Verification items for the finished model (mm, model axes). A direction names the side the tool comes from. Round coordinates to 2 decimals unless told otherwise and drop trailing zeros. Write each loop counter-clockwise with the first axis right and the second up, starting at its lowest first coordinate (ties: lowest second). Pieces come first, ordered by that corner, then holes. Notation, with made-up numbers: (4, -35) - (45, -35) arc R19 ccw to (45, -20) - close; hole circle Ø2 at (-37.75, -3). An arc over 180 degrees is marked (long way). Answer as a JSON object with one key per item and string values.
Autodesk Inventor part; units mm, degrees
ref_plane "YZ Plane" through (0, 0, 0) normal (1, 0, 0) x (0, 1, 0)
ref_plane "XZ Plane" through (0, 0, 0) normal (0, 1, 0) x (-1, 0, 0)
ref_plane "XY Plane" through (0, 0, 0) normal (0, 0, 1) x (1, 0, 0)
sketch "Skizze1" plane through (0, 0, 0) normal (0, 0, 1) x (1, 0, 0)
  line L0 (-68.45, -44.2) -> (68.45, -44.2)
  line L1 (68.45, -44.2) -> (68.45, 44.2)
  line L2 (68.45, 44.2) -> (-68.45, 44.2)
  line L3 (-68.45, 44.2) -> (-68.45, -44.2)
  line L4 (-68.45, -44.2) -> (68.45, 44.2) construction
  line L5 (68.45, -44.2) -> (-68.45, 44.2) construction
  circle A0 centre (-63.75, -39) radius 1.375
  circle A1 centre (63.75, -39) radius 1.375
  circle A2 centre (63.75, 39) radius 1.375
  circle A3 centre (-63.75, 39) radius 1.375
  line L6 (0, 61.88) -> (0, -61.88)
  line L7 (-95.83, 0) -> (95.83, 0)
  circle A4 centre (-63.75, 31.5) radius 1.375
  circle A5 centre (-63.75, -31.5) radius 1.375
  line L8 (-63.75, 39) -> (-63.75, 31.5) construction
  circle A6 centre (-11.75, 0) radius 1.375
  point P0 (0, 0)
  dimension "d0" = 136.9
  dimension "d1" = 88.4
  dimension "d2" = 2.75
  dimension "d3" = 127.5
  dimension "d4" = 78
  dimension "d7" = 63
  dimension "d8" = 2.75
  dimension "d9" = 2.75
  dimension "d10" = 52
extrude "Extrusion1" add sketch "Skizze1" along normal blind 3.6 contours L3 L7 A6 L6 L0 | L6 L7 L1 L0 | L3 L2 L6 L7 A6 | L6 L2 L1 L7
sketch "Skizze2" plane through (0, 0, 0) normal (0, 0, -1) x (-1, 0, 0)
  circle A0 centre (63.75, -31.5) radius 1.375
  circle A1 centre (63.75, 31.5) radius 1.375
  circle A2 centre (11.75, 0) radius 1.375
  line L0 (67.05, -28.2) -> (60.45, -28.2)
  line L1 (60.45, -28.2) -> (60.45, -34.8)
  line L2 (60.45, -34.8) -> (67.05, -34.8)
  line L3 (67.05, -34.8) -> (67.05, -28.2)
  line L4 (67.05, -28.2) -> (60.45, -34.8) construction
  line L5 (60.45, -28.2) -> (67.05, -34.8) construction
  line L6 (67.05, 34.8) -> (60.45, 34.8)
  line L7 (60.45, 34.8) -> (60.45, 28.2)
  line L8 (60.45, 28.2) -> (67.05, 28.2)
  line L9 (67.05, 28.2) -> (67.05, 34.8)
  circle A3 centre (63.75, 31.5) radius 1.375
  line L10 (67.05, 34.8) -> (60.45, 28.2) construction
  line L11 (60.45, 34.8) -> (67.05, 28.2) construction
  line L12 (15.05, 3.3) -> (8.45, 3.3)
  line L13 (8.45, 3.3) -> (8.45, -3.3)
  line L14 (8.45, -3.3) -> (15.05, -3.3)
  line L15 (15.05, -3.3) -> (15.05, 3.3)
  line L16 (15.05, 3.3) -> (8.45, -3.3) construction
  line L17 (8.45, 3.3) -> (15.05, -3.3) construction
  point P0 (0, 0)
  dimension "d11" = 6.6
  dimension "d12" = 6.6
extrude "Extrusion2" [suppressed]
sketch "Skizze3" plane through (0, 0, 3.6) normal (0, 0, 1) x (1, 0, 0)
  circle A0 centre (-63.75, 31.5) radius 1.375
  circle A1 centre (-63.75, -31.5) radius 1.375
  circle A2 centre (-11.75, 0) radius 1.375
  line L0 (-63.75, 31.5) -> (-63.75, -31.5) construction
  line L1 (-95.83, 0) -> (95.83, 0)
  line L2 (-67.25, -27) -> (-60.25, -27)
  line L3 (-60.25, -27) -> (-60.25, 27)
  line L4 (-60.25, 27) -> (-67.25, 27)
  line L5 (-67.25, 27) -> (-67.25, -27)
  line L6 (-67.25, -27) -> (-60.25, 27) construction
  line L7 (-60.25, -27) -> (-67.25, 27) construction
  line L8 (-52.25, -34) -> (-43.25, -34)
  line L9 (-43.25, -34) -> (-43.25, -43)
  line L10 (-43.25, -43) -> (-52.25, -43)
  line L11 (-52.25, -43) -> (-52.25, -34)
  line L12 (-34.25, -34) -> (-25.25, -34)
  line L13 (-25.25, -34) -> (-25.25, -43)
  line L14 (-25.25, -43) -> (-34.25, -43)
  line L15 (-34.25, -43) -> (-34.25, -34)
  line L16 (-47.75, -34) -> (-47.75, -43) construction
  line L17 (-29.75, -34) -> (-29.75, -43) construction
  line L18 (-52.25, -38.5) -> (-43.25, -38.5) construction
  line L19 (-27.95, 22.5) -> (-7.95, 22.5)
  line L20 (-7.95, 22.5) -> (-7.95, 42.5)
  line L21 (-7.95, 42.5) -> (-27.95, 42.5)
  line L22 (-27.95, 42.5) -> (-27.95, 22.5)
  line L23 (-17.95, 42.5) -> (-17.95, 22.5) construction
  point P0 (0, 0)
  point P1 (-63.75, 0)
  dimension "d15" = 7
  dimension "d16" = 54
  dimension "d17" = 9
  dimension "d18" = 9
  dimension "d19" = 9
  dimension "d20" = 18
  dimension "d21" = 16
  dimension "d22" = 7
  dimension "d23" = 20
  dimension "d25" = 11
  dimension "d26" = 20
  dimension "d29" = 45.8
extrude "Extrusion3" cut sketch "Skizze3" against normal blind 3 contours L3 L2 L5 L1 | L1 L5 L4 L3 | L8 L9 L10 L11 | L12 L13 L14 L15 | L22 L21 L20 L19
sketch "Skizze4" plane through (0, 0, 3.6) normal (0, 0, 1) x (1, 0, 0)
  line L0 (-31.95, 18.5) -> (-17.75, 18.5)
  line L1 (-17.75, 18.5) -> (-17.75, -30)
  line L2 (-17.75, -30) -> (-56.25, -30)
  line L3 (-56.25, -30) -> (-56.25, 38.5)
  line L4 (-31.95, 18.5) -> (-31.95, 38.5)
  line L5 (-31.95, 38.5) -> (-56.25, 38.5)
  line L6 (-1.95, 35) -> (58.05, 35)
  line L7 (58.05, 35) -> (58.05, -35)
  line L8 (58.05, -35) -> (-1.95, -35)
  line L9 (-1.95, -35) -> (-1.95, 35)
  line L10 (-7.95, 22.5) -> (-27.95, 22.5)
  line L11 (-7.95, 42.5) -> (-7.95, 22.5)
  line L12 (-27.95, 42.5) -> (-7.95, 42.5)
  line L13 (-27.95, 22.5) -> (-27.95, 42.5)
  line L14 (-60.25, -27) -> (-67.25, -27)
  line L15 (-60.25, 27) -> (-60.25, -27)
  line L16 (-67.25, 27) -> (-60.25, 27)
  line L17 (-67.25, -27) -> (-67.25, 27)
  line L18 (-34.25, -34) -> (-25.25, -34)
  line L19 (-34.25, -43) -> (-34.25, -34)
  line L20 (-25.25, -43) -> (-34.25, -43)
  line L21 (-25.25, -34) -> (-25.25, -43)
  circle A0 centre (-11.75, 0) radius 1.375
  line L22 (-95.83, 0) -> (95.83, 0)
  line L23 (0, 61.88) -> (0, -61.88)
  point P0 (0, 0)
  dimension "d30" = 4
  dimension "d31" = 4
  dimension "d32" = 4
  dimension "d34" = 4
  dimension "d35" = 6
  dimension "d36" = 4
  dimension "d37" = 6
  dimension "d38" = 70
  dimension "d39" = 60
extrude "Extrusion4" cut sketch "Skizze4" against normal blind 2 contours L9 L6 L23 L22 | L22 L23 L8 L9 | L0 L1 L22 L3 L5 L4 | L1 L2 L3 L22 | L23 L6 L7 L22 | L22 L7 L8 L23
sketch "Skizze5" plane through (0, 0, 3.6) normal (0, 0, 1) x (1, 0, 0)
  circle A0 centre (-63.75, 39) radius 1.375
  circle A1 centre (-63.75, -39) radius 1.375
  circle A2 centre (63.75, -39) radius 1.375
  circle A3 centre (63.75, 39) radius 1.375
  line L0 (-67.25, 43) -> (-60.25, 43)
  line L1 (-60.25, 43) -> (-60.25, 36)
  line L2 (-60.25, 36) -> (-67.25, 36)
  line L3 (-67.25, 36) -> (-67.25, 43)
  line L4 (-67.25, -43) -> (-60.25, -43)
  line L5 (-60.25, -43) -> (-60.25, -36)
  line L6 (-60.25, -36) -> (-67.25, -36)
  line L7 (-67.25, -36) -> (-67.25, -43)
  line L8 (60.25, 36) -> (67.25, 36)
  line L9 (67.25, 36) -> (67.25, 43)
  line L10 (67.25, 43) -> (60.25, 43)
  line L11 (60.25, 43) -> (60.25, 36)
  circle A4 centre (63.75, 39) radius 1.375
  line L12 (60.25, -43) -> (67.25, -43)
  line L13 (67.25, -43) -> (67.25, -36)
  line L14 (67.25, -36) -> (60.25, -36)
  line L15 (60.25, -36) -> (60.25, -43)
  line L16 (0, 61.88) -> (0, -61.88)
  line L17 (-95.83, 0) -> (95.83, 0)
  line L18 (-63.75, 36) -> (-63.75, 43) construction
  line L19 (3.5, -43) -> (-3.5, -43)
  line L20 (-3.5, -43) -> (-3.5, -36)
  line L21 (-3.5, -36) -> (3.5, -36)
  line L22 (3.5, -36) -> (3.5, -43)
  line L23 (3.5, 36) -> (-3.5, 36)
  line L24 (-3.5, 36) -> (-3.5, 43)
  line L25 (-3.5, 43) -> (3.5, 43)
  line L26 (3.5, 43) -> (3.5, 36)
  point P0 (0, 0)
  dimension "d42" = 7
  dimension "d46" = 3
  dimension "d47" = 4
  dimension "d51" = 7
extrude "Extrusion5" add sketch "Skizze5" along normal blind 20.2
sketch "Skizze7" plane through (0, 0, 23.8) normal (0, 0, 1) x (1, 0, 0)
  line L0 (-3.5, -43) -> (3.5, -43)
  line L1 (3.5, -43) -> (3.5, -36)
  line L2 (3.5, -36) -> (-3.5, -36)
  line L3 (-3.5, -36) -> (-3.5, -43)
  point P0 (0, 0)
extrude "Extrusion7" cut sketch "Skizze7" against normal blind 3.2
fillet "Rundung1" radius 2 8 edges at (-60.25, 36, 13.7) (-60.25, -36, 13.7) (60.25, 36, 13.7) (60.25, -36, 13.7) (3.5, -36, 12.1) (3.5, 36, 13.7) (-3.5, 36, 13.7) (-3.5, -36, 12.1)
sketch "Skizze6" plane through (0, 0, 3.6) normal (0, 0, 1) x (1, 0, 0)
  line L0 (-60.25, 43) -> (-67.25, 43)
  line L1 (-67.25, 43) -> (-67.25, 36)
  line L2 (67.25, -43) -> (67.25, -36)
  line L3 (60.25, -43) -> (67.25, -43)
  line L4 (-67.25, 43) -> (67.25, 43)
  line L5 (67.25, 43) -> (67.25, -43)
  line L6 (67.25, -43) -> (-67.25, -43)
  line L7 (-67.25, -43) -> (-67.25, 43)
  line L8 (68.45, 44.2) -> (-68.45, 44.2)
  line L9 (-68.45, 44.2) -> (-68.45, -44.2)
  line L10 (-68.45, -44.2) -> (68.45, -44.2)
  line L11 (68.45, -44.2) -> (68.45, 44.2)
  point P0 (0, 0)
  dimension "d48" = 1.2
extrude "Extrusion6" add sketch "Skizze6" along normal blind 22
sketch "Skizze8" plane through (-68.45, 44.2, 0) normal (0, 1, 0) x (1, 0, 0)
  line L0 (68.45, 3.96) -> (68.45, -23.76)
  line L1 (164.28, 0) -> (-27.38, 0)
  line L2 (19.2, -4) -> (8.2, -4)
  line L3 (8.2, -4) -> (8.2, -9)
  line L4 (8.2, -9) -> (19.2, -9)
  line L5 (19.2, -9) -> (19.2, -4)
  line L6 (19.2, -4) -> (8.2, -9) construction
  line L7 (8.2, -4) -> (19.2, -9) construction
  line L8 (58.55, -5.2) -> (42.35, -5.2)
  line L9 (42.35, -5.2) -> (42.35, -19.8)
  line L10 (42.35, -19.8) -> (58.55, -19.8)
  line L11 (58.55, -19.8) -> (58.55, -5.2)
  line L12 (58.55, -5.2) -> (42.35, -19.8) construction
  line L13 (42.35, -5.2) -> (58.55, -19.8) construction
  line L14 (42.35, -5.2) -> (37.35, -5.2)
  line L15 (37.35, -5.2) -> (37.35, -6.7)
  line L16 (37.35, -6.7) -> (42.35, -10.8955)
  line L17 (19.2, -9) -> (21.7, -6.5)
  line L18 (21.7, -6.5) -> (19.2, -4)
  line L19 (21.7, -6.5) -> (13.7, -6.5) construction
  point P0 (68.45, 0)
  point P1 (50.45, -12.5)
  dimension "d55" = 54.75
  dimension "d56" = 6.5
  dimension "d57" = 11
  dimension "d58" = 5
  dimension "d61" = 18
  dimension "d63" = 14.6
  dimension "d64" = 16.2
  dimension "d65" = 5.2
  dimension "d66" = 50
  dimension "d67" = 1.5
  dimension "d68" = 5
  dimension "d69" = 2.5
extrude "Extrusion8" cut sketch "Skizze8" against normal up to surface (1.2 mm away)
sketch "Skizze9" plane through (-68.45, -44.2, 0) normal (0, -1, 0) x (1, 0, 0)
  line L0 (0, 0) -> (136.9, 0)
  line L1 (136.9, 0) -> (136.9, 25.6)
  line L2 (0, 25.6) -> (136.9, 25.6)
  line L3 (0, 0) -> (0, 25.6)
  line L4 (135.7, 25.6) -> (1.2, 25.6)
  line L5 (8.2, 25.6) -> (64.95, 25.6)
  line L6 (64.95, 25.6) -> (64.95, 5.6)
  line L7 (64.95, 5.6) -> (8.2, 5.6)
  line L8 (8.2, 5.6) -> (8.2, 25.6)
  line L9 (16.2, 3.6) -> (25.2, 3.6)
  line L10 (16.2, 3.6) -> (16.2, 0.6)
  line L11 (16.2, 0.6) -> (25.2, 0.6)
  line L12 (25.2, 3.6) -> (25.2, 0.6)
  line L13 (34.2, 3.6) -> (43.2, 3.6)
  line L14 (34.2, 3.6) -> (34.2, 0.6)
  line L15 (34.2, 0.6) -> (43.2, 0.6)
  line L16 (43.2, 3.6) -> (43.2, 0.6)
  line L17 (16.2, 0.6) -> (25.2, 0.6) construction
  line L18 (20.7, 0.6) -> (20.7, 3.6) construction
  line L19 (34.2, 0.6) -> (43.2, 0.6) construction
  line L20 (38.7, 0.6) -> (38.7, 3.6) construction
  line L21 (8.2, 23.8) -> (8.2, 3.6)
  line L22 (8.2, 3.6) -> (8.2, 23.8)
  point P0 (68.45, 0)
  dimension "d73" = 64.95
  dimension "d75" = 2
extrude "Extrusion9" cut sketch "Skizze9" against normal up to surface (1.2 mm away) contours L2 L6 L7 L8
fillet "Rundung2" radius 3 8 edges at (-68.45, -44.2, 12.8) (-68.45, 44.2, 12.8) (68.45, -44.2, 12.8) (68.45, 44.2, 12.8) (67.25, 43, 24.7) (67.25, -43, 24.7) (-67.25, -43, 24.7) (-67.25, 43, 24.7)
fillet "Rundung3" radius 1 6 edges at (-26.1, 43.6, 10.8955) (-49.25, 43.6, 9) (-49.25, 43.6, 4) (-46.75, 43.6, 6.5) (-60.25, 43.6, 9) (-60.25, 43.6, 4)
equation "\"d9\" = d8"
equation "\"d18\" = d17"
equation "\"d51\" = d42"
properties part number "Gehaeuse BS v3" material "PC/ABS-Kunststoff"
1. Cross-section at C-C (x = -21). Record the boundary of the cut face in (y, z).
Completed:
{"outline": "(-44.2, 0) - (44.2, 0) - (44.2, 5.2) - (43, 5.2) - (43, 3.6) - (42.5, 3.6) - (42.5, 0.6) - (22.5, 0.6) - (22.5, 3.6) - (18.5, 3.6) - (18.5, 1.6) - (-30, 1.6) - (-30, 3.6) - (-43, 3.6) - (-43, 5.6) - (-44.2, 5.6) - close; (43, 19.8) - (44.2, 19.8) - (44.2, 25.6) - (43, 25.6) - close"}
2. Material ranges on probe 1 along Y at (x, z) = (63.75, 18.5) (3 decimals); probe 2 along X at (y, z) = (40.5, 18.5); probe 3 along Y at (x, z) = (-63.75, 0.8) (3 decimals), recorded low to high. Write a range as from..to.
Completed:
{"probe 1": "y = -44.2..-40.375, -37.625..-36, 36..37.625, 40.375..44.2", "probe 2": "x = -68.45..-60.25, -3.5..3.5, 60.25..68.45", "probe 3": "y = -44.2..-40.375, -37.625..-32.875, -30.125..-27, 27..30.125, 32.875..37.625, 40.375..44.2"}
3. Access from +Z, -Z, +X, -X, +Y, -Y to the whole of each face (thin tool, end or side, straight path). Record for faces 1 (the face through (66.35, -42.14, 24.71)), 2 (the face through (-63.01, 30.34, 1.77)).
Completed:
{"face 1": "+Z", "face 2": "+Z, -Z"}
4. Cross-section at A-A (z = 18). Count the separate pieces of the cut face and the enclosed holes in it, plus the area to 3 significant figures.
Completed:
{"separate pieces": "2", "enclosed holes": "4", "area": "703 mm^2"}
5. Cross-section at D-D (x = 38). Record the boundary of the cut face in (y, z), plus the area to 3 significant figures.
Completed:
{"outline": "(-44.2, 0) - (44.2, 0) - (44.2, 25.6) - (43, 25.6) - (43, 3.6) - (35, 3.6) - (35, 1.6) - (-35, 1.6) - (-35, 3.6) - (-43, 3.6) - (-43, 25.6) - (-44.2, 25.6) - close", "area": "231 mm^2"}
6. Go/stop test with flat-tipped pins: pin 1 (1.6 mm diameter, centred on x = -63.75, y = 39, fed in from -Z); pin 2 (4 mm diameter, centred on y = -41.5, z = 11, fed in from -X); pin 3 (2 mm diameter, centred on x = -65, y = -38, fed in from +Z); pin 4 (10 mm diameter, centred on x = -14, z = 18.5, fed in from -Y). Record where each tip stops, or that it passes through.
Completed:
{"pin 1": "passes through", "pin 2": "stops at x = -68.45", "pin 3": "stops at z = 23.8", "pin 4": "stops at y = 43"}
7. Cross-section at B-B (y = 31.5). Record the boundary of the cut face in (x, z) (3 decimals), plus the area to 3 significant figures.
Completed:
{"outline": "(-68.45, 0) - (-65.125, 0) - (-65.125, 3.6) - (-67.25, 3.6) - (-67.25, 25.6) - (-68.45, 25.6) - close; (-62.375, 0) - (68.45, 0) - (68.45, 25.6) - (67.25, 25.6) - (67.25, 3.6) - (58.05, 3.6) - (58.05, 1.6) - (-1.95, 1.6) - (-1.95, 3.6) - (-7.95, 3.6) - (-7.95, 0.6) - (-27.95, 0.6) - (-27.95, 3.6) - (-31.95, 3.6) - (-31.95, 1.6) - (-56.25, 1.6) - (-56.25, 3.6) - (-62.375, 3.6) - close", "area": "307 mm^2"}
